Autodesk Inventor part; units mm, degrees
ref_plane "YZ Plane" through (0, 0, 0) normal (1, 0, 0) x (0, 1, 0)
ref_plane "XZ Plane" through (0, 0, 0) normal (0, 1, 0) x (-1, 0, 0)
ref_plane "XY Plane" through (0, 0, 0) normal (0, 0, 1) x (1, 0, 0)
sketch "Skizze1" plane through (0, 0, 0) normal (0, 1, 0) x (-1, 0, 0)
  circle A0 centre (0, 0) radius 6
  dimension "d0" = 12
extrude "Extrusion1" add sketch "Skizze1" along normal blind 11
sketch "Skizze2" plane through (0, 0, 0) normal (0, -1, 0) x (1, 0, 0)
  circle A0 centre (0, 0) radius 4
  dimension "d3" = 8
extrude "Extrusion2" add sketch "Skizze2" against normal blind 19
sketch "Skizze3" plane through (0, 0, 0) normal (0, -1, 0) x (1, 0, 0)
  circle A0 centre (0, 0) radius 15
  dimension "d6" = 30
extrude "Extrusion3" add sketch "Skizze3" along normal blind 6
sketch "Skizze4" plane through (0, -6, 0) normal (0, -1, 0) x (1, 0, 0)
  point P0 (0, 0)
  point P1 (10, 0)
  dimension "d9" = 10
hole "Bohrung1" at (10, -6, 0) direction (0, 1, 0) diameter 3.4 end through all
pattern_circular "Runde Anordnung1" count 4 over 360 about axis through (0, 0, 0) along (0, -1, 0) of "Bohrung1"
properties part number "dynamixel_pro_frame_shaft"
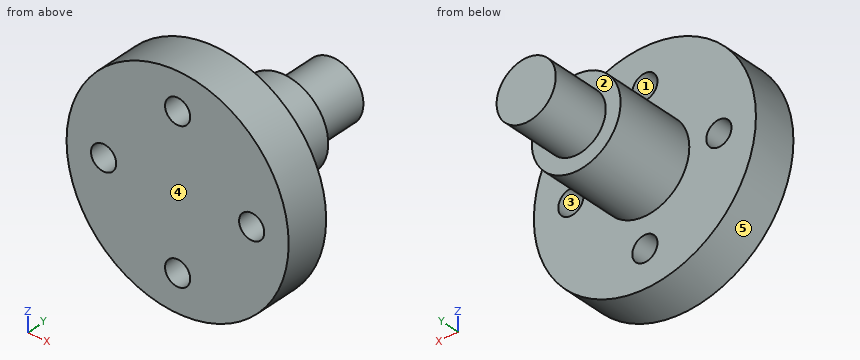
Part model, mm, in its own coordinate system. Face numbers are marked on the shaded views. A direction names the side the tool comes from. Coordinates: 2 decimals unless noted, no trailing zeros. Loops run counter-clockwise (first coordinate to the right, second up) from the corner with the lowest first, then second, coordinate; pieces in that order, holes last. Notation, with made-up numbers: M -35.75,15 L -31.75,15 A34 ccw -31.75,45 Z; hole C 45,78.25 d1. An arc over 180 degrees is marked long. Use a Markdown table: item, result. Add a question column.
Q1. Probe L1, parallel to Z at x = 0, y = -1.55; L2, parallel to X at y = -3.5, z = 11.25; L3, parallel to Y at x = 1, z = 12.5. List the from-to ranges inside material, lowest first.
Q2. Pin check, flat tips, straight feed: P1, Ø4, axis at x = 0, z = -10, coming from the +Y side; P2, Ø3, axis at x = 10.5, y = -0.5, coming from the +Z side; P3, Ø10, axis at y = -2.5, z = -8.5, coming from the +X side. Stop position of each tip, or through.
Q3. Which spindle directions (+Z, -Z, +X, -X, +Y, -Y) get a long thin tool onto all of the face, cutting with end or side? Do the marked faces 1 and 2. Say none if no direction does.
Q4. Mould opens along X. For the marked faces 3, 4 and 5 say: +X half, -X half, draft (parallel to the pull), parting line (faces both ways), or undercut.
Q5. Cut at B-B (y = -1.75). Write the cut outline in (x, z).
Q6. Cut at A-A (z = 0). Write the cut outline in (x, y), and give its area (3 significant figures).
Q7. Cut at C-C (x = 0). Write the cut outline in (y, z).
Q8. Cut at D-D (x = -9.25). Write the cut outline in (y, z).
Worked out:
| question | item | result |
|---|---|---|
| 1 | L1 | z = -15 to -11.7, -8.3 to 8.3, 11.7 to 15 |
| 1 | L2 | x = -9.92 to -1.15, 1.15 to 9.92 |
| 1 | L3 | y = -6 to 0 |
| 2 | P1 | stops at y = 0 |
| 2 | P2 | stops at z = 12 |
| 2 | P3 | stops at x = 14.59 |
| 3 | face 1 | +Y, -Y |
| 3 | face 2 | +Y |
| 4 | face 3 | undercut |
| 4 | face 4 | draft |
| 4 | face 5 | parting line |
| 5 | outline | C 0,0 d30; hole C -10,0 d3.4; hole C 0,-10 d3.4; hole C 0,10 d3.4; hole C 10,0 d3.4 |
| 6 | outline | M -15,-6 L -11.7,-6 L -11.7,0 L -15,0 Z; M -8.3,-6 L 8.3,-6 L 8.3,0 L 6,0 L 6,11 L 4,11 L 4,19 L -4,19 L -4,11 L -6,11 L -6,0 L -8.3,0 Z; M 11.7,-6 L 15,-6 L 15,0 L 11.7,0 Z |
| 6 | area | 335 mm2 |
| 7 | outline | M -6,-15 L 0,-15 L 0,-11.7 L -6,-11.7 Z; M -6,-8.3 L 0,-8.3 L 0,-6 L 11,-6 L 11,-4 L 19,-4 L 19,4 L 11,4 L 11,6 L 0,6 L 0,8.3 L -6,8.3 Z; M -6,11.7 L 0,11.7 L 0,15 L -6,15 Z |
| 8 | outline | M -6,-11.81 L 0,-11.81 L 0,-1.53 L -6,-1.53 Z; M -6,1.53 L 0,1.53 L 0,11.81 L -6,11.81 Z |
